from build123d import *

# Parameters (mm, degrees)
F0_R     = 28.575
F1_DEPTH = 40.2336
F2_R     = 10.16
F3_DEPTH = 15.7734
F4_R     = 3.302


# Not quite as in the source:
# - a feature names something its author has since deleted; it is built from what else it names


with BuildPart() as f1:
    # F0 (on Top) → F1 (new body)
    with BuildSketch(Plane.XY):
        Circle(F0_R)
        with BuildLine():
            ThreePointArc((-13.4477648793, 4.826), (0, 14.2875), (13.4477648793, 4.826))
            Line((13.4477648793, 4.826), (18.5293, 4.826))
            Line((18.5293, 4.826), (18.5293, -4.826))
            Line((18.5293, -4.826), (13.4477648793, -4.826))
            ThreePointArc((13.4477648793, -4.826), (0, -14.2875), (-13.4477648793, -4.826))
            Line((-13.4477648793, -4.826), (-18.5293, -4.826))
            Line((-18.5293, -4.826), (-18.5293, 4.826))
            Line((-18.5293, 4.826), (-13.4477648793, 4.826))
        make_face(mode=Mode.SUBTRACT)
        with BuildLine():
            ThreePointArc((-13.4477648793, -4.826), (-14.2875, 0), (-13.4477648793, 4.826))
            Line((-13.4477648793, 4.826), (-18.5293, 4.826))
            Line((-18.5293, 4.826), (-18.5293, -4.826))
            Line((-18.5293, -4.826), (-13.4477648793, -4.826))
        make_face()
    extrude(amount=F1_DEPTH)

    # F2 (on Top) → F3 (join)
    with BuildSketch(Plane.XY):
        with BuildLine():
            ThreePointArc((57.2172352941, -19.4161565532), (68.9970276056, -12.7215530348), (73.66, 0))
            ThreePointArc((73.66, 0), (68.9970276056, 12.7215530348), (57.2172352941, 19.4161565532))
            ThreePointArc((57.2172352941, 19.4161565532), (34.29, 0), (57.2172352941, -19.4161565532))
        make_face()
        with Locations((53.975, 0)):
            Circle(F2_R, mode=Mode.SUBTRACT)
        with BuildLine():
            ThreePointArc((57.2172352941, -19.4161565532), (34.29, 0), (57.2172352941, 19.4161565532))
            Line((57.2172352941, 19.4161565532), (4.7064705882, 28.1847433836))
            ThreePointArc((4.7064705882, 28.1847433836), (21.8061691049, 18.4667705344), (28.575, 0))
            ThreePointArc((28.575, 0), (21.8061691049, -18.4667705344), (4.7064705882, -28.1847433836))
            Line((4.7064705882, -28.1847433836), (57.2172352941, -19.4161565532))
        make_face()
    extrude(amount=F3_DEPTH)

    # F4
    f4_edges = [f1.edges().sort_by_distance(p)[0] for p in [
        (-28.575, 0, 40.2336),
    ]]
    fillet(f4_edges, radius=F4_R)


solid = f1.part
Here's how the part is built. I have some questions about the finished solid (model axes, mm). A direction names the side the tool comes from. Coordinates: 2 decimals unless noted, no trailing zeros. Order: outer loops, then holes, each group sorted by start corner. A loop starts at its lowest first (then second) coordinate and runs counter-clockwise, first axis right, second up.
Item 1: I need wall thicknesses on line 1 (X direction, y = 0.5, z = 13); line 2 (X direction, y = 25, z = 38); line 3 (Y direction, x = -6.5, z = 10). Which ranges of each line are inside material? Lowest first, please.
Result sheet:
line 1: x = -28.57 to -14.28, 18.53 to 43.83, 64.12 to 73.65
line 2: x = -13.47 to 13.47
line 3: y = -27.83 to -12.72, 12.72 to 27.83
Item 2: For P1, Ø8, axis at x = 32.5, y = -13, coming from the +Z side; P2, Ø2.5, axis at x = 15, z = 22.5, coming from the +Y side; P3, Ø2, axis at x = 51, z = 11.5, coming from the -Y side; P4, Ø8, axis at x = 57.5, y = 0, coming from the -Z side, each with a flat end and sliding along its axis, tell me the tip position at first contact or that it passes through.
Result sheet:
P1: stops at z = 15.77
P2: stops at y = 25.05
P3: stops at y = -20.62
P4: passes through
Item 3: If we section it at C-C on z = 8: State how many separate pieces and enclosed holes the cut face has, plus the area to 3 significant figures.
Result sheet:
separate pieces: 1
enclosed holes: 2
area: 3,520 mm2
Item 4: If we section it at A-A on y = 0: List the corners of the cut face in (x, z) for me (1 decimal), plus the area to 3 significant figures.
Result sheet:
outline: (-28.6, 0) - (-14.3, 0) - (-14.3, 40.2) - (-25.3, 40.2) arc R3.3 ccw to (-28.6, 36.9) - close; (18.5, 0) - (43.8, 0) - (43.8, 15.8) - (28.6, 15.8) - (28.6, 36.9) arc R3.3 ccw to (25.3, 40.2) - (18.5, 40.2) - close; (64.1, 0) - (73.7, 0) - (73.7, 15.8) - (64.1, 15.8) - close
area: 1,360 mm2
Item 5: For faces 1 (the face through (16, -4.826, 20)), 2 (the face through (11, -11, 40.234)), 3 (the face through (-28.547, 1.256, 22.311)), which set-ups out of +Z, -Z, +X, -X, +Y, -Y let a thin tool reach every point of the face, with its end or its side?
Result sheet:
face 1: +Z, -Z
face 2: +Z, +X, -X, +Y, -Y
face 3: +Z
Item 6: If we section it at B-B on x = 0: List the corners of the cut face in (y, z) for me (1 decimal), plus the area to 3 significant figures.
Result sheet:
outline: (-28.6, 0) - (-14.3, 0) - (-14.3, 40.2) - (-25.3, 40.2) arc R3.3 ccw to (-28.6, 36.9) - close; (14.3, 0) - (28.6, 0) - (28.6, 36.9) arc R3.3 ccw to (25.3, 40.2) - (14.3, 40.2) - close
area: 1,140 mm2
Item 7: If we mould it in two halves opening along Y, with no side actions, what happens to faces 4 (the face through (31.33, 23.74, 7.78)), 5 (the face through (18.529, 0, 20)), 6 (the face through (16, 4.826, 20)), 7 (the face through (73.656, -0.387, 7.776))? For each: +Y half, -Y half, draft (parallel to the pull), parting line (faces both ways), or undercut.
Result sheet:
face 4: +Y half
face 5: undercut
face 6: undercut
face 7: parting line
